from build123d import *

# Parameters (mm, degrees)
CROQUIS1_W              = 10
CROQUIS1_H              = 3
CROQUIS1_W_2            = 3
CROQUIS1_H_2            = 10
CROQUIS1_W_3            = 7
CROQUIS1_W_4            = 8
CROQUIS1_H_3            = 8
SALIENTE_EXTRUIR1_DEPTH = 3
SKETCH1_W               = 12
SKETCH1_H               = 25
SKETCH1_W_2             = 18
SKETCH1_H_2             = 66
CUT_EXTRUDE2_DEPTH      = 10


with BuildPart() as part:
    # Croquis1 → Saliente-Extruir1 (new body)
    with BuildSketch(Plane(origin=(0, 0, 0), x_dir=(1, 0, 0), z_dir=(0, 1, 0))):
        Polygon((17.5, 79), (20.5, 79), (20.5, 80), (25.626440042, 80), (30, 80), (30, 83), (40, 83), (40, 80), (50, 80), (50, 83), (60, 83), (60, 80), (70, 80), (70, 83), (80, 83), (80, 80), (84.373559958, 80), (89.5, 80), (89.5, 79), (92.5, 79), (92.5, 74), (89.5, 74), (89.5, 69), (92.5, 69), (92.5, 65), (107, 65), (107, 68), (117.5, 68), (117.5, 65), (132.5, 65), (132.5, 68), (147.5, 68), (147.5, 65), (162.5, 65), (162.5, 68), (177.5, 68), (177.5, 65), (192.5, 65), (192.5, 68), (207.5, 68), (207.5, 65), (222.5, 65), (222.5, 68), (237.5, 68), (237.5, 65), (252.5, 65), (252.5, 68), (260, 68), (260, 82.5), (257, 82.5), (257, 97.5), (260, 97.5), (260, 112.5), (257, 112.5), (257, 127.5), (260, 127.5), (260, 142.5), (257, 142.5), (257, 157.5), (260, 157.5), (260, 172.5), (257, 172.5), (257, 187.5), (260, 187.5), (260, 202.5), (257, 202.5), (257, 217.5), (260, 217.5), (260, 232.5), (257, 232.5), (257, 247.5), (260, 247.5), (260, 265), (242.5, 265), (242.5, 262), (227.5, 262), (227.5, 265), (212.5, 265), (212.5, 262), (197.5, 262), (197.5, 265), (182.5, 265), (182.5, 262), (167.5, 262), (167.5, 265), (152.5, 265), (152.5, 262), (137.5, 262), (137.5, 265), (122.5, 265), (122.5, 262), (107.5, 262), (107.5, 265), (92.5, 265), (92.5, 262), (77.5, 262), (77.5, 155), (77.5, 140), (3, 140), (0, 140), (0, 125), (3, 125), (3, 110), (0, 110), (0, 95), (3, 95), (3, 80), (0, 80), (0, 65), (17.5, 65), (17.5, 69), (20.5, 69), (20.5, 74), (17.5, 74), align=None)
        with Locations((120, 141.5)):
            Rectangle(CROQUIS1_W, CROQUIS1_H, mode=Mode.SUBTRACT)
        Polygon((120, 93), (70, 93), (70, 116), (170, 116), (170, 93), align=None, mode=Mode.SUBTRACT)
        with Locations((200, 141.5)):
            Rectangle(CROQUIS1_W, CROQUIS1_H, mode=Mode.SUBTRACT)
        with Locations((96.5, 151.5)):
            Rectangle(CROQUIS1_W_2, CROQUIS1_H_2, mode=Mode.SUBTRACT)
        with Locations((96.5, 131.5)):
            Rectangle(CROQUIS1_W_2, CROQUIS1_H_2, mode=Mode.SUBTRACT)
        with Locations((101.5, 141.5)):
            Rectangle(CROQUIS1_W_3, CROQUIS1_H, mode=Mode.SUBTRACT)
        with Locations((143.5, 151.5)):
            Rectangle(CROQUIS1_W_2, CROQUIS1_H_2, mode=Mode.SUBTRACT)
        with Locations((143.5, 131.5)):
            Rectangle(CROQUIS1_W_2, CROQUIS1_H_2, mode=Mode.SUBTRACT)
        with Locations((176.5, 151.5)):
            Rectangle(CROQUIS1_W_2, CROQUIS1_H_2, mode=Mode.SUBTRACT)
        with Locations((138.5, 141.5)):
            Rectangle(CROQUIS1_W_3, CROQUIS1_H, mode=Mode.SUBTRACT)
        with Locations((181.5, 141.5)):
            Rectangle(CROQUIS1_W_3, CROQUIS1_H, mode=Mode.SUBTRACT)
        with Locations((223.5, 151.5)):
            Rectangle(CROQUIS1_W_2, CROQUIS1_H_2, mode=Mode.SUBTRACT)
        with Locations((218.5, 141.5)):
            Rectangle(CROQUIS1_W_3, CROQUIS1_H, mode=Mode.SUBTRACT)
        with Locations((176.5, 131.5)):
            Rectangle(CROQUIS1_W_2, CROQUIS1_H_2, mode=Mode.SUBTRACT)
        with Locations((223.5, 131.5)):
            Rectangle(CROQUIS1_W_2, CROQUIS1_H_2, mode=Mode.SUBTRACT)
        with Locations((93.5, 248)):
            Rectangle(CROQUIS1_W_4, CROQUIS1_H_3, mode=Mode.SUBTRACT)
        with Locations((146.5, 248)):
            Rectangle(CROQUIS1_W_4, CROQUIS1_H_3, mode=Mode.SUBTRACT)
        with Locations((173.5, 248)):
            Rectangle(CROQUIS1_W_4, CROQUIS1_H_3, mode=Mode.SUBTRACT)
        with Locations((226.5, 248)):
            Rectangle(CROQUIS1_W_4, CROQUIS1_H_3, mode=Mode.SUBTRACT)
    extrude(amount=SALIENTE_EXTRUIR1_DEPTH)

    # Sketch1 → Cut-Extrude2 (cut)
    with BuildSketch(Plane.XZ):
        with Locations((241, -194)):
            Rectangle(SKETCH1_W, SKETCH1_H)
        with Locations((219, -194)):
            Rectangle(SKETCH1_W_2, SKETCH1_H_2)
    extrude(amount=-CUT_EXTRUDE2_DEPTH, mode=Mode.SUBTRACT)


solid = part.part
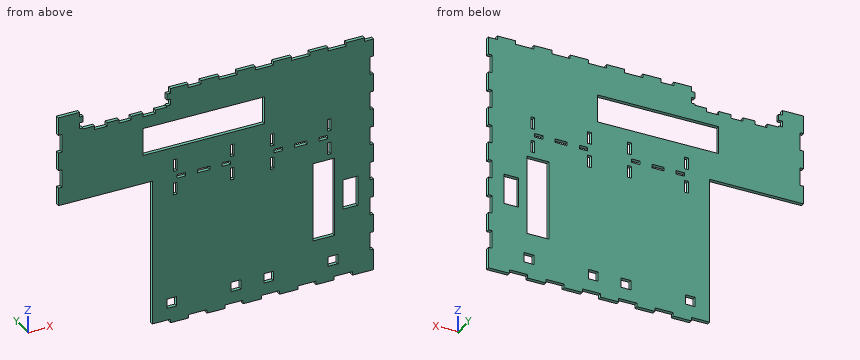
Could you check a few things on this model? Use its own coordinates, in mm. Give positions to 0.01 mm unless a question says otherwise; leave off trailing zeros. Write each loop counter-clockwise with the first axis right and the second up, starting at its lowest first coordinate (ties: lowest second). Pieces come first, ordered by that corner, then holes. Notation, with made-up numbers: (62.5, -20) - (95.5, -20) arc R8 ccw to (95.5, -16) - close; hole circle Ø8 at (-2.5, -11.5). An arc over 180 degrees is marked (long way). Use CSV: the item, a comma, the result in double quotes. Start each with the question number.
Item 1: If I drill on line 1 along X through (y, z) = (1.05, -184); line 2 along X through (y, z) = (2.2, -194.5); line 3 along Z through (x, y) = (149.5, 2.2), over which ranges is the centre line in solid material (lowest first)?
Item 2: I want a section at C-C, the plane x = 66.5. Please give me the cut outline in (y, z).
Item 3: I want a section at A-A, the plane z = -169. Please give me the cut outline in (x, y), then the cut area to 4 significant figures.
Item 4: I'm going to push flat-ended pins straight in: pin 1 (0.9 mm diameter, centred on y = 2, z = -239.5, fed in from +X); pin 2 (0.9 mm diameter, centred on x = 176.5, y = 1, fed in from -Z); pin 3 (0.9 mm diameter, centred on y = 1, z = -67, fed in from +X). Where does each tip first touch, or does it pass through?
Item 5: I want a section at B-B, the plane z = -104. Please give me the cut outline in (x, y).
Item 6: I want a section at D-D, the plane y = 1.75. Give the number of separate pieces and of enclosed holes in the cut face, then the cut area to 3 significant figures.
Findings:
1,line 1,"x = 77.5 to 210, 228 to 235, 247 to 257"
1,line 2,"x = 77.5 to 210, 228 to 235, 247 to 260"
1,line 3,"z = -262 to -252, -244 to -116, -93 to -65"
2,outline,"(0, -140) - (3, -140) - (3, -80) - (0, -80) - close"
3,outline,"(77.5, 0) - (210, 0) - (210, 3) - (77.5, 3) - close; (228, 0) - (260, 0) - (260, 3) - (228, 3) - close"
3,area,"493.5 mm2"
4,pin 1,"stops at x = 257"
4,pin 2,"stops at z = -262"
4,pin 3,"stops at x = 252.5"
5,outline,"(0, 0) - (70, 0) - (70, 3) - (0, 3) - close; (170, 0) - (260, 0) - (260, 3) - (170, 3) - close"
6,separate pieces,"1"
6,enclosed holes,"21"
6,area,"35,800 mm2"
